```python
from build123d import *

# Parameters (mm, degrees)
SKETCH1_R           = 4
BOSS_EXTRUDE1_DEPTH = 5
SKETCH2_R           = 5.5
SKETCH2_R_2         = 4
BOSS_EXTRUDE2_DEPTH = 5


with BuildPart() as part:
    # Sketch1 → Boss-Extrude1 (new body)
    with BuildSketch(Plane.XY):
        with BuildLine():
            Line((-6.5, 3.741657387), (-6.5, -3.741657387))
            ThreePointArc((-6.5, -3.741657387), (0, -7.5), (6.5, -3.741657387))
            Line((6.5, -3.741657387), (6.5, 3.741657387))
            ThreePointArc((6.5, 3.741657387), (0, 7.5), (-6.5, 3.741657387))
        make_face()
        Circle(SKETCH1_R, mode=Mode.SUBTRACT)
    extrude(amount=BOSS_EXTRUDE1_DEPTH)

    # Sketch2 → Boss-Extrude2 (add)
    with BuildSketch(Plane(origin=(0, 0, 0), x_dir=(-1, 0, 0), z_dir=(0, 0, -1))):
        Circle(SKETCH2_R)
        Circle(SKETCH2_R_2, mode=Mode.SUBTRACT)
    extrude(amount=BOSS_EXTRUDE2_DEPTH)


solid = part.part
```
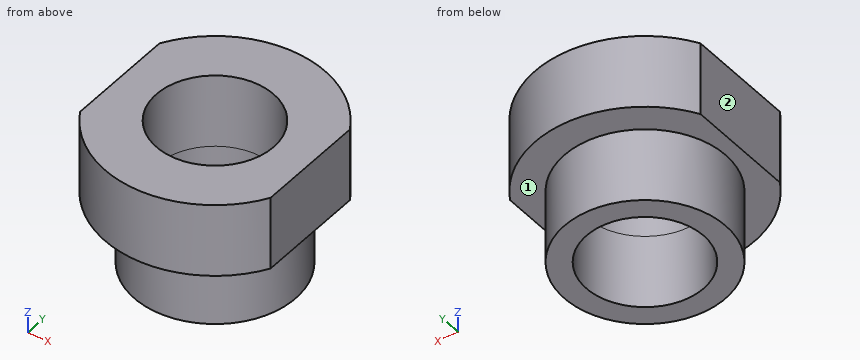
Build history of the part. All positions in model axes, mm. Face numbers are marked on the shaded views. A direction names the side the tool comes from. Round coordinates to 2 decimals unless told otherwise and drop trailing zeros. Write each loop counter-clockwise with the first axis right and the second up, starting at its lowest first coordinate (ties: lowest second). Pieces come first, ordered by that corner, then holes.
1) Band-saw the part on B-B, the plane x = 0. List the corners of the cut face in (y, z), and give its area (3 significant figures).
2) Drill centre lines: probe 1 along X at (y, z) = (0, 3.1); probe 2 along Y at (x, z) = (0, -3.75); probe 3 along Y at (x, z) = (-1.75, -3.5). Where is each one in solid material? Low to high.
3) Band-saw the part on D-D, the plane x = 4.25. List the corners of the cut face in (y, z), and give its area (3 significant figures).
4) Pin check, flat tips, straight feed: pin 1 (1 mm diameter, centred on y = 4, z = -3, fed in from +X); pin 2 (6.5 mm diameter, centred on x = 0, y = 0, fed in from -Z). Stop position of each tip, or through.
5) 3-axis set-ups, long thin cutter, end or side, ignore diameter. For the marked faces 1 and 2: which of +Z, -Z, +X, -X, +Y, -Y reach the whole face in a straight line?
6) Band-saw the part on A-A, the plane y = 0. List the corners of the cut face in (x, z).
7) Band-saw the part on C-C, the plane z = 2.75. List the corners of the cut face in (x, y), and give its area (3 significant figures).
Ans:
1. outline: (-7.5, 0) - (-5.5, 0) - (-5.5, -5) - (-4, -5) - (-4, 5) - (-7.5, 5) - close; (4, -5) - (5.5, -5) - (5.5, 0) - (7.5, 0) - (7.5, 5) - (4, 5) - close
1. area: 50.0 mm2
2. probe 1: x = -6.5 to -4, 4 to 6.5
2. probe 2: y = -5.5 to -4, 4 to 5.5
2. probe 3: y = -5.21 to -3.6, 3.6 to 5.21
3. outline: (-6.18, 0) - (-3.49, 0) - (-3.49, -5) - (3.49, -5) - (3.49, 0) - (6.18, 0) - (6.18, 5) - (-6.18, 5) - close
3. area: 96.7 mm2
4. pin 1: stops at x = 4.24
4. pin 2: passes through
5. face 1: -Z
5. face 2: +Z, -Z, -X, +Y, -Y
6. outline: (-6.5, 0) - (-5.5, 0) - (-5.5, -5) - (-4, -5) - (-4, 5) - (-6.5, 5) - close; (4, -5) - (5.5, -5) - (5.5, 0) - (6.5, 0) - (6.5, 5) - (4, 5) - close
7. outline: (-6.5, -3.74) arc R7.5 ccw to (6.5, -3.74) - (6.5, 3.74) arc R7.5 ccw to (-6.5, 3.74) - close; hole circle Ø8 at (0, 0)
7. area: 116 mm2
